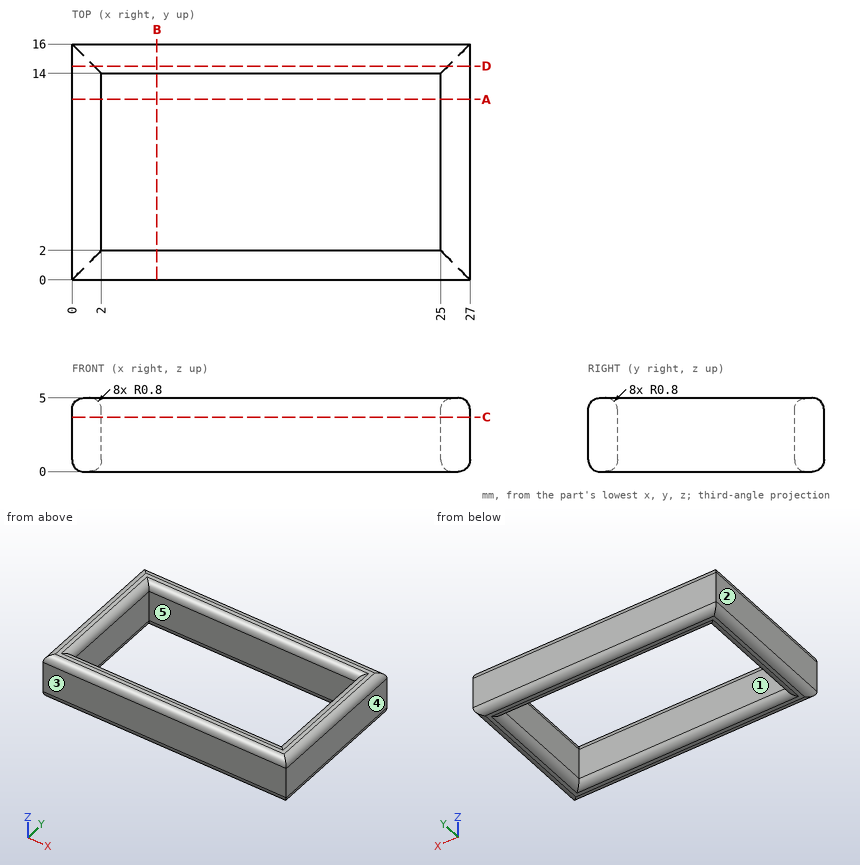
Answer from the drawing. Dimensions are ordinates in mm from the lowest x, y and z of the part. A direction names the side the tool comes from. Round coordinates to 2 decimals unless told otherwise and drop trailing zeros. Write each loop counter-clockwise with the first axis right and the second up, starting at its lowest first coordinate (ties: lowest second). Pieces come first, ordered by that corner, then holes.
1. Straight lines are drawn through the part: L1, parallel to X at y = 10.25, z = 2.55; L2, parallel to Y at x = 24.25, z = 2.3; L3, parallel to Z at x = 1.75, y = 15.25. For each, find the intervals that lie inside material, in ascending order.
2. The part is cut by section D-D, the plane y = 14.5. Determine the outline of the cut face in (x, z), then the cut area to 3 significant figures.
3. Determine the mould class of the marked faces 3, 4 and 5 for opening direction Y: pulls with the +Y half, pulls with the -Y half, needs draft (parallel to the pull), parting line crosses it, or undercut.
4. The part is cut by section C-C, the plane z = 3.7. Determine the outline of the cut face in (x, y).
5. The part is cut by section B-B, the plane x = 5.75. Determine the outline of the cut face in (y, z), then the cut area to 3 significant figures.
6. Which of the six approach directions +Z, -Z, +X, -X, +Y, -Y give full straight-line access (tool end or side, diameter ignored) to the marked faces 1 and 2?
7. The part is cut by section A-A, the plane y = 12.25. Determine the outline of the cut face in (x, z).
Values:
1. L1: x = 0 to 2, 25 to 27
1. L2: y = 0 to 2, 14 to 16
1. L3: z = 0 to 5
2. outline: (0, 0.8) arc R0.8 ccw to (0.8, 0) - (1.2, 0) arc R0.8 ccw to (1.5, 0.06) - (25.5, 0.06) arc R0.8 ccw to (25.8, 0) - (26.2, 0) arc R0.8 ccw to (27, 0.8) - (27, 4.2) arc R0.8 ccw to (26.2, 5) - (25.8, 5) arc R0.8 ccw to (25.5, 4.94) - (1.5, 4.94) arc R0.8 ccw to (1.2, 5) - (0.8, 5) arc R0.8 ccw to (0, 4.2) - close
2. area: 132 mm2
3. face 3: pulls with the -Y half
3. face 4: needs draft
3. face 5: undercut
4. outline: (0, 0) - (27, 0) - (27, 16) - (0, 16) - close; hole (2, 2) - (25, 2) - (25, 14) - (2, 14) - close
5. outline: (0, 0.8) arc R0.8 ccw to (0.8, 0) - (1.2, 0) arc R0.8 ccw to (2, 0.8) - (2, 4.2) arc R0.8 ccw to (1.2, 5) - (0.8, 5) arc R0.8 ccw to (0, 4.2) - close; (14, 0.8) arc R0.8 ccw to (14.8, 0) - (15.2, 0) arc R0.8 ccw to (16, 0.8) - (16, 4.2) arc R0.8 ccw to (15.2, 5) - (14.8, 5) arc R0.8 ccw to (14, 4.2) - close
5. area: 18.9 mm2
6. face 1: +Z, -Z
6. face 2: +Z, -Z, -X, +Y, -Y
7. outline: (0, 0.8) arc R0.8 ccw to (0.8, 0) - (1.2, 0) arc R0.8 ccw to (2, 0.8) - (2, 4.2) arc R0.8 ccw to (1.2, 5) - (0.8, 5) arc R0.8 ccw to (0, 4.2) - close; (25, 0.8) arc R0.8 ccw to (25.8, 0) - (26.2, 0) arc R0.8 ccw to (27, 0.8) - (27, 4.2) arc R0.8 ccw to (26.2, 5) - (25.8, 5) arc R0.8 ccw to (25, 4.2) - close
